Check sheet for the modelled part. Datum: model origin and axes. Units: mm. A direction names the side the tool comes from. Round coordinates to 2 decimals unless told otherwise and drop trailing zeros. Write each loop counter-clockwise with the first axis right and the second up, starting at its lowest first coordinate (ties: lowest second). Pieces come first, ordered by that corner, then holes. Notation, with made-up numbers: (-24.5, 51) -> (3.5, 51) arc R32 ccw to (3.5, 79) -> close; hole circle Ø11 at (85.25, 44.25). An arc over 180 degrees is marked (long way). Answer as a JSON object with one key per item and string values. Group by question number.
Autodesk Inventor part; units mm, degrees
ref_plane "YZ Plane" through (0, 0, 0) normal (1, 0, 0) x (0, 1, 0)
ref_plane "XZ Plane" through (0, 0, 0) normal (0, 1, 0) x (-1, 0, 0)
ref_plane "XY Plane" through (0, 0, 0) normal (0, 0, 1) x (1, 0, 0)
sketch "Sketch1" plane through (0, 0, 0) normal (0, 1, 0) x (-1, 0, 0)
  line L0 (-3.4641, 0) -> (-1.7321, 3)
  line L1 (-1.7321, 3) -> (1.7321, 3)
  line L2 (1.7321, 3) -> (3.4641, 0)
  line L3 (3.4641, 0) -> (1.7321, -3)
  line L4 (1.7321, -3) -> (-1.7321, -3)
  line L5 (-1.7321, -3) -> (-3.4641, 0)
  point P0 (0, 0)
  point P1 (0, 0)
  dimension "d1" = 6
extrude "Extrusion1" add sketch "Sketch1" along normal blind 50
sketch "Sketch2" plane through (0, 0, 0) normal (0, -1, 0) x (1, 0, 0)
  circle A0 centre (0, 0) radius 1.75
  dimension "d4" = 3.5
sketch "Sketch3" plane through (0, 50, 0) normal (0, 1, 0) x (1, 0, 0)
  circle A0 centre (0, 0) radius 1.5
  dimension "d5" = 3
extrude "Extrusion2" add sketch "Sketch3" along normal blind 6.31
extrude "Extrusion3" cut sketch "Sketch2" against normal blind 6
thread "Thread1"
thread "Thread2"
properties part number "spacer5cm"
(1) Go/stop test with flat-tipped pins: pin 1 Ø1.5 at (x, z) = (-1.5, 1.5) entering from +Y; pin 2 Ø1.5 at (y, z) = (21, -1.5) entering from +X; pin 3 Ø1.8 at (x, z) = (0, 0) entering from -Y. Record where each tip stops, or that it passes through.
(2) Section check B-B on y = 33. Record the cut outline in (x, z).
(3) Section check C-C on z = -2.45. Record the cut outline in (x, y).
(4) Section check D-D on y = 51. Record the cut outline in (x, z).
(5) Section check A-A on x = 0. Record the cut outline in (y, z), then the cut area to 3 significant figures.
(6) Release check for a two-part mould opening along X. For faces 4 (the flat face through (0, 25, 3)), 5 (the cylindrical face through (1.617, 2.958, -0.67)), 6 (the flat face through (2.6, 24.6, -1.5)) record: pulls with the +X half, pulls with the -X half, needs draft (parallel to the pull), parting line crosses it, or undercut.
(7) Access from +Z, -Z, +X, -X, +Y, -Y to the whole of each face (thin tool, end or side, straight path). Record for faces 1 (the flat face through (2.6, 24.6, 1.5)), 2 (the flat face through (0, 6, 0)), 3 (the flat face through (-1.5, 50, 0.7)).
(8) Scan lines: line 1 along Z through (x, y) = (0, 4.05); line 2 along Y through (x, z) = (-1.75, -0.65); line 3 along X through (y, z) = (35.5, 0.8). Record each from-to range of solid material in increasing order.
Data:
{
 "1": {"pin 1": "stops at y = 56.31", "pin 2": "stops at x = 3.03", "pin 3": "stops at y = 6"},
 "2": {"outline": "(-3.46, 0) -> (-1.73, -3) -> (1.73, -3) -> (3.46, 0) -> (1.73, 3) -> (-1.73, 3) -> close"},
 "3": {"outline": "(-2.05, 0) -> (2.05, 0) -> (2.05, 50) -> (-2.05, 50) -> close"},
 "4": {"outline": "circle Ø3 at (0, 0)"},
 "5": {"outline": "(0, -3) -> (50, -3) -> (50, -1.5) -> (56.31, -1.5) -> (56.31, 1.5) -> (50, 1.5) -> (50, 3) -> (0, 3) -> (0, 1.75) -> (6, 1.75) -> (6, -1.75) -> (0, -1.75) -> close", "area": "298 mm²"},
 "6": {"face 4": "needs draft", "face 5": "undercut", "face 6": "pulls with the +X half"},
 "7": {"face 1": "+Z, +X, +Y, -Y", "face 2": "-Y", "face 3": "+Y"},
 "8": {"line 1": "z = -3 to -1.75, 1.75 to 3", "line 2": "y = 0 to 50", "line 3": "x = -3 to 3"}
}
